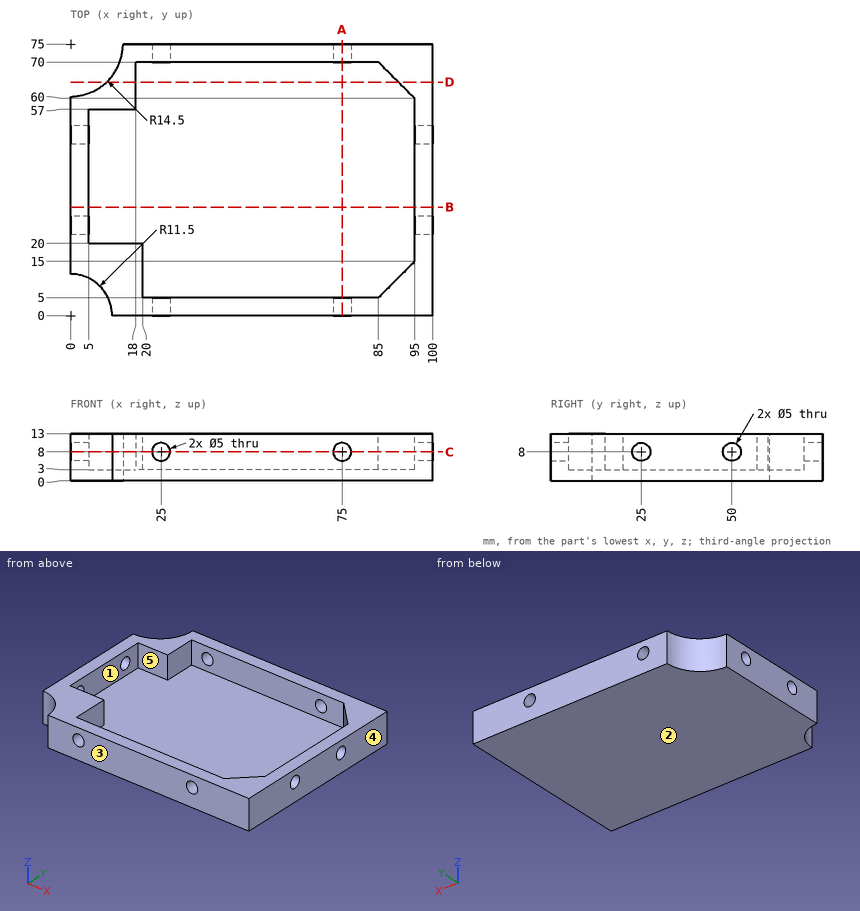
Verification items for this drawing (mm, ordinates from the low corner). A direction names the side the tool comes from. Coordinates: 2 decimals unless noted, no trailing zeros. Loops run counter-clockwise (first coordinate to the right, second up) from the corner with the lowest first, then second, coordinate; pieces in that order, holes last.
Item 1: Release check for a two-part mould opening along X. For the marked faces 3, 4 and 5 record: released by +X, released by -X, zero draft, split by the parting line, or undercut.
Item 2: Sectioned sample at A-A, the plane x = 75. Record the boundary of the cut face in (y, z), then the cut area to 3 significant figures.
Item 3: Sectioned sample at D-D, the plane y = 64.5. Record the boundary of the cut face in (x, z), then the cut area to 3 significant figures.
Item 4: Go/stop test with flat-tipped pins: pin 1 Ø3 at (y, z) = (25, 8) entering from +X; pin 2 Ø3 at (x, z) = (10, 8.5) entering from +Y; pin 3 Ø8 at (x, y) = (73.5, 52) entering from +Z. Record where each tip stops, or that it passes through.
Item 5: Sectioned sample at C-C, the plane z = 8. Count the separate pieces of the cut face and the enclosed holes in it, then the cut area to 4 significant figures.
Item 6: Thickness scan on line 1 (Z direction, x = 98.5, y = 50); line 2 (Y direction, x = 46, z = 6); line 3 (X direction, y = 15, z = 5.25). Record the ranges inside material, lowest first.
Item 7: Sectioned sample at B-B, the plane y = 30. Record the boundary of the cut face in (x, z), then the cut area to 3 significant figures.
Item 8: Access from +Z, -Z, +X, -X, +Y, -Y to the whole of each face (thin tool, end or side, straight path). Record for the marked faces 1 and 2.
Check result:
1. face 3: zero draft
1. face 4: released by +X
1. face 5: undercut
2. outline: (0, 0) - (75, 0) - (75, 5.5) - (70, 5.5) - (70, 3) - (5, 3) - (5, 5.5) - (0, 5.5) - close; (0, 10.5) - (5, 10.5) - (5, 13) - (0, 13) - close; (70, 10.5) - (75, 10.5) - (75, 13) - (70, 13) - close
2. area: 275 mm2
3. outline: (10, 0) - (100, 0) - (100, 13) - (90.5, 13) - (90.5, 3) - (18, 3) - (18, 13) - (10, 13) - close
3. area: 445 mm2
4. pin 1: passes through
4. pin 2: stops at y = 66.17
4. pin 3: stops at z = 3
5. separate pieces: 8
5. enclosed holes: 0
5. area: 1,675 mm2
6. line 1: z = 0 to 5.5, 10.5 to 13
6. line 2: y = 0 to 5, 70 to 75
6. line 3: x = 0 to 20, 95 to 100
7. outline: (0, 0) - (100, 0) - (100, 13) - (95, 13) - (95, 3) - (5, 3) - (5, 13) - (0, 13) - close
7. area: 400 mm2
8. face 1: +Z
8. face 2: -Z, +X, -X, +Y, -Y
